Can you work these out from the model? Positions are in its coordinate system, mm. A direction names the side the tool comes from. Give positions to 0.01 mm unless a question says otherwise; leave off trailing zeros. Order: outer loops, then holes, each group sorted by start corner. A loop starts at its lowest first (then second) coordinate and runs counter-clockwise, first axis right, second up.
```python
from build123d import *

# Parameters (mm, degrees)
SKETCH1_R             = 66.675
BOSS_EXTRUDE1_DEPTH   = 6.35
BOSS_EXTRUDE2_REACH   = 240.306
CIRPATTERN1_COUNT     = 3
CUT_EXTRUDE1_DEPTH    = 118.618
CIRPATTERN2_COUNT     = 3
CUT_EXTRUDE2_DEPTH    = 12.7
CIRPATTERN3_COUNT     = 3
HOLE1_D               = 4.0386
CIRPATTERN4_OUTLINE_R = 2.0193
CIRPATTERN4_DEPTH     = 6.35
HOLE2_D               = 9.525
FILLET1_R             = 1.5875
HOLE3_D               = 6.985
CIRPATTERN5_COUNT     = 3
HOLE5_D               = 3.7973
CIRPATTERN6_COUNT     = 3
CIRPATTERN7_COUNT     = 3


# Read off the part's stored shape, not the designer's step: CirPattern4
with BuildPart() as part:
    # Sketch1 → Boss-Extrude1 (new body)
    with BuildSketch(Plane(origin=(0, 0, 0), x_dir=(1, 0, 0), z_dir=(0, 1, 0))):
        with Locations(Location((0, 0, 0), (0, 0, 270))):
            Circle(SKETCH1_R)
    extrude(amount=BOSS_EXTRUDE1_DEPTH)

    # Sketch2 → Boss-Extrude2 (add, up to next)
    with BuildSketch(Plane(origin=(0, 124.968, -124.968), x_dir=(1, 0, 0), z_dir=(0, -1, 0)), mode=Mode.PRIVATE) as boss_extrude2_sk1:
        with BuildLine():
            Line((-29.614770643, 184.705098882), (-8.635999998, 172.593000013))
            Line((-8.635999998, 172.593000013), (8.636000002, 172.593000013))
            Line((8.636000002, 172.593000013), (29.61477065, 184.705098878))
            ThreePointArc((29.61477065, 184.705098878), (4e-09, 191.642999985), (-29.614770643, 184.705098882))
        make_face()
    boss_extrude2_tool1 = extrude(boss_extrude2_sk1.sketch, amount=BOSS_EXTRUDE2_REACH, mode=Mode.PRIVATE) - part.part
    boss_extrude2 = boss_extrude2_tool1.solids().sort_by_distance((0, 124.968, 57.682703))[0]
    add(boss_extrude2)

    # CirPattern1: Boss-Extrude2 ×3 about axis
    cirpattern1_axis = Axis((0, 0, 0), (0, 1, 0))
    for i in range(1, CIRPATTERN1_COUNT):
        add(boss_extrude2.rotate(cirpattern1_axis, i * 360 / CIRPATTERN1_COUNT))

    # Sketch4 → Cut-Extrude1 (cut)
    with BuildSketch(Plane(origin=(0, 124.968, 0), x_dir=(1, 0, 0), z_dir=(0, 1, 0))):
        Polygon((14.575202222, -51.054000013), (11.527202222, -56.333290875), (5.588000002, -52.904290875), (8.636000002, -47.625000013), align=None)
        Polygon((-14.575202225, -51.054000007), (-8.635999998, -47.625000013), (-5.587999998, -52.904290875), (-11.527202221, -56.333290877), align=None)
    cut_extrude1 = extrude(amount=-CUT_EXTRUDE1_DEPTH, mode=Mode.SUBTRACT)

    # CirPattern2: Cut-Extrude1 ×3 about axis
    cirpattern2_axis = Axis((0, 0, 0), (0, 1, 0))
    for i in range(1, CIRPATTERN2_COUNT):
        add(cut_extrude1.rotate(cirpattern2_axis, i * 360 / CIRPATTERN2_COUNT), mode=Mode.SUBTRACT)

    # Sketch5 → Cut-Extrude2 (cut)
    with BuildSketch(Plane(origin=(0, 124.968, 0), x_dir=(1, 0, 0), z_dir=(0, 1, 0))):
        with BuildLine():
            Line((29.61477065, -59.737098878), (26.275063747, -57.808918214))
            ThreePointArc((26.275063747, -57.808918214), (-4e-09, -63.5), (-26.275063755, -57.808918211))
            Line((-26.275063755, -57.808918211), (-29.614770643, -59.737098882))
            ThreePointArc((-29.614770643, -59.737098882), (4e-09, -66.674999985), (29.61477065, -59.737098878))
        make_face()
    cut_extrude2 = extrude(amount=-CUT_EXTRUDE2_DEPTH, mode=Mode.SUBTRACT)

    # CirPattern3: Cut-Extrude2 ×3 about axis
    cirpattern3_axis = Axis((0, 0, 0), (0, 1, 0))
    for i in range(1, CIRPATTERN3_COUNT):
        add(cut_extrude2.rotate(cirpattern3_axis, i * 360 / CIRPATTERN3_COUNT), mode=Mode.SUBTRACT)

    # Hole1 (through all)
    with Locations(Plane(origin=(0, 0, 0), x_dir=(-1, 0, 0), z_dir=(0, -1, 0))):
        with Locations((-19.05, 53.975), (19.05, 53.975)):
            Hole(HOLE1_D / 2)

    # CirPattern4 outline → CirPattern4 (cut)
    with BuildSketch(Plane(origin=(0, 0, 0), x_dir=(1, 0, 0), z_dir=(0, 1, 0))):
        with Locations((-37.218721169, -43.485283942)):
            Circle(CIRPATTERN4_OUTLINE_R)
        with Locations((-56.268721169, -10.489716058)):
            Circle(CIRPATTERN4_OUTLINE_R)
        with Locations((56.268721169, -10.489716058)):
            Circle(CIRPATTERN4_OUTLINE_R)
        with Locations((37.218721169, -43.485283942)):
            Circle(CIRPATTERN4_OUTLINE_R)
    extrude(amount=CIRPATTERN4_DEPTH, mode=Mode.SUBTRACT)

    # Hole2 (through all)
    with Locations(Plane(origin=(0, 6.35, 0), x_dir=(1, 0, 0), z_dir=(0, 1, 0))):
        with Locations((0, 0)):
            Hole(HOLE2_D / 2)

    # Fillet1
    fillet1_edges = [part.edges().sort_by_distance(p)[0] for p in [
        (4.7625, 6.35, 0),
        (4.7625, 0, 0),
    ]]
    fillet(fillet1_edges, radius=FILLET1_R)

    # Hole3 (through all)
    with Locations(Plane(origin=(0, 6.35, 0), x_dir=(1, 0, 0), z_dir=(0, 1, 0))):
        with Locations((0, 19.05), (0, -19.05)):
            Hole(HOLE3_D / 2)

    # Sketch19 → Hole4 (revolve, cut)
    with BuildSketch(Plane(origin=(-50.350429877, 124.968, -28.940765488), x_dir=(0, 0, 1), z_dir=(1, 0, 0))):
        Polygon((0, 0), (0, 7.525163199), (1.9558, 6.35), (1.9558, 3.175), (2.3622, 3.175), (2.3622, 0), align=None)
    hole4 = revolve(axis=Axis((-50.350429877, 131.318, -28.940765488), (0, -1, 0)), mode=Mode.SUBTRACT)

    # CirPattern5: Hole4 ×3 about axis
    cirpattern5_axis = Axis((0, 0, 0), (0, 1, 0))
    for i in range(1, CIRPATTERN5_COUNT):
        add(hole4.rotate(cirpattern5_axis, i * 360 / CIRPATTERN5_COUNT), mode=Mode.SUBTRACT)

    # Hole5 (through all)
    with Locations(Plane(origin=(0, 6.35, 0), x_dir=(1, 0, 0), z_dir=(0, 1, 0))):
        with Locations((-29.972, 53.975), (29.972, 53.975)):
            hole5 = Hole(HOLE5_D / 2)

    # CirPattern6: Hole5 ×3 about axis
    cirpattern6_axis = Axis((0, 0, 0), (0, 1, 0))
    for i in range(1, CIRPATTERN6_COUNT):
        add(hole5.rotate(cirpattern6_axis, i * 360 / CIRPATTERN6_COUNT), mode=Mode.SUBTRACT)

    # Sketch23 → Hole6 (revolve, cut)
    with BuildSketch(Plane(origin=(0, 124.968, 51.435), x_dir=(0, 0, 1), z_dir=(1, 0, 0))):
        Polygon((0, 0), (0, 5.239163199), (1.9558, 4.064), (1.9558, 3.175), (2.3622, 3.175), (2.3622, 0), align=None)
    hole6 = revolve(axis=Axis((0, 131.318, 51.435), (0, -1, 0)), mode=Mode.SUBTRACT)

    # CirPattern7: Hole6 ×3 about axis
    cirpattern7_axis = Axis((0, 0, 0), (0, 1, 0))
    for i in range(1, CIRPATTERN7_COUNT):
        add(hole6.rotate(cirpattern7_axis, i * 360 / CIRPATTERN7_COUNT), mode=Mode.SUBTRACT)


solid = part.part
```
1) Suppose I cut it at C-C (z = 19.05). Please give me the cut outline in (x, y).
2) If I drill on line 1 (Z direction, x = 0, y = 2) (1 decimal); line 2 (Y direction, x = -40.5, z = 46.5); line 3 (X direction, y = 3, z = 0) (1 decimal), over which ranges is the centre line in solid material (lowest first)?
3) Suppose I cut it at B-B (x = -19.05). Please give me the cut outline in (y, z), and give its area (3 significant figures).
4) We'd pull the mould along Z, two halves only. Please class faces 4 (the face through (36.926, 66, -47)), 5 (the face through (47.065, 66.489, -18.936)), 6 (the face through (-42.635, 121.355, -26.141)): +Z half, -Z half, draft (parallel to the pull), parting line (faces both ways), or undercut.
5) Which directions (+Z, -Z, +X, -X, +Y, -Y) give clear straight access to the entire face, cutting with the end or side of a thin tool? Please do faces 1 (the face through (-1.878, 3.131, 16.105)), 2 (the face through (41.305, 66.489, -23.708)), 3 (the face through (51.54, 66.49, -19.92)).
6) Suppose I cut it at D-D (z = -58). Please give me the cut outline in (x, y), and give its area (3 significant figures).
7) Suppose I cut it at A-A (y = 85). Give the number of separate pieces and of enclosed holes in the cut face, and give its area (3 significant figures).
8) I'm going to push flat-ended pins straight in: pin 1 Ø3 at (x, z) = (-18, 4) entering from -Y; pin 2 Ø5 at (x, y) = (0, 68.5) entering from -Z (3 decimals); pin 3 Ø3.5 at (x, z) = (-37.22, 43.49) entering from -Y; pin 4 Ø1 at (x, y) = (-37.5, 42) entering from -Z. Where does each tip first touch, or does it pass through?
Results:
1. outline: (-63.9, 0) - (-3.49, 0) - (-3.49, 6.35) - (-63.9, 6.35) - close; (3.49, 0) - (63.9, 0) - (63.9, 6.35) - (3.49, 6.35) - close
2. line 1: z = -66.7 to -22.5, -15.6 to -4.8, 4.8 to 15.6, 22.5 to 66.7
2. line 2: y = 0 to 6.35
2. line 3: x = -66.7 to -63.3, -60.1 to -4.8, 4.8 to 60.1, 63.3 to 66.7
3. outline: (0, -63.9) - (6.35, -63.9) - (6.35, -55.99) - (0, -55.99) - close; (0, -51.96) - (6.35, -51.96) - (6.35, 53.64) - (124.97, 53.64) - (124.97, 60.58) - (112.27, 60.58) - (112.27, 63.9) - (0, 63.9) - close
3. area: 1,960 mm2
4. face 4: draft
4. face 5: +Z half
4. face 6: undercut
5. face 1: +Y, -Y
5. face 2: +Z, +Y
5. face 3: +Y
6. outline: (-32.89, 0) - (32.89, 0) - (32.89, 6.35) - (-32.89, 6.35) - close
6. area: 418 mm2
7. separate pieces: 3
7. enclosed holes: 0
7. area: 1,970 mm2
8. pin 1: stops at y = 0
8. pin 2: stops at z = 47.625
8. pin 3: passes through
8. pin 4: stops at z = -55.47
